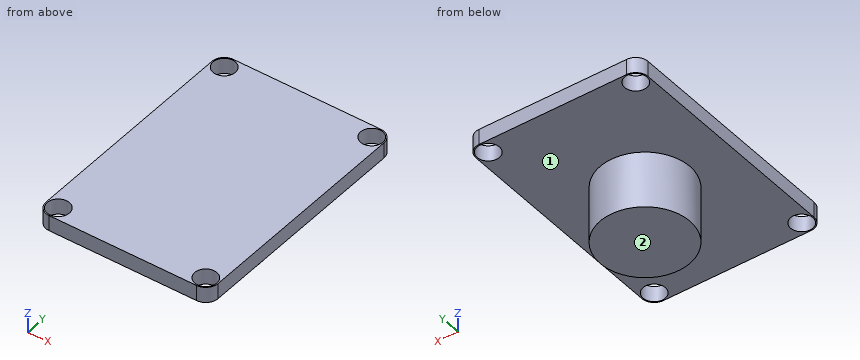
from build123d import *

# Parameters (mm, degrees)
SKETCH2_R           = 1.156401536
BOSS_EXTRUDE1_DEPTH = 1.6256
SKETCH3_R           = 4.65455
BOSS_EXTRUDE2_DEPTH = 5.8801


with BuildPart() as part:
    # Sketch2 → Boss-Extrude1 (new body)
    with BuildSketch(Plane.XY):
        with BuildLine():
            Line((-7.6581, -12.7889), (7.6581, -12.7889))
            ThreePointArc((7.6581, -12.7889), (8.556125612, -12.416925612), (8.9281, -11.5189))
            Line((8.9281, -11.5189), (8.9281, 11.5189))
            ThreePointArc((8.9281, 11.5189), (8.556125612, 12.416925612), (7.6581, 12.7889))
            Line((7.6581, 12.7889), (-7.6581, 12.7889))
            ThreePointArc((-7.6581, 12.7889), (-8.556125612, 12.416925612), (-8.9281, 11.5189))
            Line((-8.9281, 11.5189), (-8.9281, -11.5189))
            ThreePointArc((-8.9281, -11.5189), (-8.556125612, -12.416925612), (-7.6581, -12.7889))
        make_face()
        with Locations((7.6581, 11.5189)):
            Circle(SKETCH2_R, mode=Mode.SUBTRACT)
        with Locations((-7.6581, 11.5189)):
            Circle(SKETCH2_R, mode=Mode.SUBTRACT)
        with Locations((7.6581, -11.5189)):
            Circle(SKETCH2_R, mode=Mode.SUBTRACT)
        with Locations((-7.6581, -11.5189)):
            Circle(SKETCH2_R, mode=Mode.SUBTRACT)
    extrude(amount=BOSS_EXTRUDE1_DEPTH)

    # Sketch3 → Boss-Extrude2 (add)
    with BuildSketch(Plane(origin=(0, 0, 0), x_dir=(-1, 0, 0), z_dir=(0, 0, -1))):
        Circle(SKETCH3_R)
    extrude(amount=BOSS_EXTRUDE2_DEPTH)


solid = part.part
Part model, mm, in its own coordinate system. Face numbers are marked on the shaded views. A direction names the side the tool comes from. Coordinates: 2 decimals unless noted, no trailing zeros. Order: outer loops, then holes, each group sorted by start corner. A loop starts at its lowest first (then second) coordinate and runs counter-clockwise, first axis right, second up.
(1) Slice it at C-C, the plane y = 0. Write the cut outline in (x, z), and give its area (3 significant figures).
Check sheet entries:
outline: (-8.93, 0) - (-4.65, 0) - (-4.65, -5.88) - (4.65, -5.88) - (4.65, 0) - (8.93, 0) - (8.93, 1.63) - (-8.93, 1.63) - close
area: 83.8 mm2
(2) Pin check, flat tips, straight feed: pin 1 Ø2.5 at (x, y) = (-7.66, -11.52) entering from -Z; pin 2 Ø4 at (y, z) = (0, -4) entering from +X. Stop position of each tip, or through.
Check sheet entries:
pin 1: stops at z = 0
pin 2: stops at x = 4.65
(3) Slice it at B-B, the plane x = -7. Write the cut outline in (y, z), and give its area (3 significant figures).
Check sheet entries:
outline: (-12.79, 0) - (-12.47, 0) - (-12.47, 1.63) - (-12.79, 1.63) - close; (-10.57, 0) - (10.57, 0) - (10.57, 1.63) - (-10.57, 1.63) - close; (12.47, 0) - (12.79, 0) - (12.79, 1.63) - (12.47, 1.63) - close
area: 35.4 mm2
(4) Probe L1, parallel to Z at x = -6.5, y = 2.5; L2, parallel to X at y = -1, z = -1.5; L3, parallel to Y at x = 3.5, z = -3. List the from-to ranges inside material, lowest first.
Check sheet entries:
L1: z = 0 to 1.63
L2: x = -4.55 to 4.55
L3: y = -3.07 to 3.07
(5) Slice it at A-A, the plane x = 0. Write the cut outline in (y, z), and give its area (3 significant figures).
Check sheet entries:
outline: (-12.79, 0) - (-4.65, 0) - (-4.65, -5.88) - (4.65, -5.88) - (4.65, 0) - (12.79, 0) - (12.79, 1.63) - (-12.79, 1.63) - close
area: 96.3 mm2
(6) Tool access for the marked faces 1 and 2: list every direction of +Z, -Z, +X, -X, +Y, -Y with a clear straight run to the whole face (end or side of a thin tool).
Check sheet entries:
face 1: -Z
face 2: -Z, +X, -X, +Y, -Y
(7) Slice it at D-D, the plane z = -4.75. Write the cut outline in (x, y), and give its area (3 significant figures).
Check sheet entries:
outline: circle Ø9.31 at (0, 0)
area: 68.1 mm2
